Source: CAD feature listing. Evaluate the final solid. Frame: model axes, mm. Round coordinates to 2 decimals unless told otherwise and drop trailing zeros. Order: outer loops, then holes, each group sorted by start corner. A loop starts at its lowest first (then second) coordinate and runs counter-clockwise, first axis right, second up. Notation, with made-up numbers: (11, 8.5) -> (47, 8.5) arc R29 cw to (47, 42.5) -> close; hole circle Ø8 at (-12, -34). An arc over 180 degrees is marked (long way). Answer as CSV lines item,"result". Start each with the question number.
(1) Section query A-A (x = -82). Output: boundary loops of the cut face in (y, z), plus the area to 3 significant figures.
(2) Section query D-D (z = 1.5). Count the separate pieces of the cut face and the enclosed holes in it, plus the area to 3 significant figures.
(3) Section query C-C (x = -98). Output: boundary loops of the cut face in (y, z), plus the area to 3 significant figures.
(4) Contact query for flat-ended pins moving along their axis: P1, Ø1.8, axis at x = -69.58, y = -54.6, coming from the +Z side; P2, Ø3, axis at y = -96, z = 1, coming from the +X side; P3, Ø1, axis at x = -31.5, z = -1, coming from the +Y side; P4, Ø2, axis at x = -53.5, z = 0, coming from the +Y side. Output: stop coordinate, or through.
(5) Line query: line 1 along Y through (x, z) = (0, -0.8) (3 decimals); line 2 along X through (y, z) = (-65, -0.15); line 3 along Y through (x, z) = (-26.5, 1.15). Output: solid intervals per line, ascending. Write a range as from..to.
(6) Section query B-B (x = -54). Output: boundary loops of the cut face in (y, z).
```python
from build123d import *

# Parameters (mm, degrees)
SKETCH_1_R               = 18.5
SKETCH_1_R_2             = 1.525
SKETCH_1_R_3             = 3
EXTRUDE_1_DEPTH          = 2.5
SKETCH_4_R               = 1.525
CUT_EXTRUDE_3_DEPTH      = 10
PATTERN_CIRCULAR_2_COUNT = 6
SKETCH_5_R               = 1.525
CUT_EXTRUDE_4_DEPTH      = 31.54
CUT_EXTRUDE_5_DEPTH      = 31.54
EXTRUDE_2_DEPTH          = 5
EXTRUDE_3_DEPTH          = 5
FILLET_2_R               = 1.5
FILLET_2_2_R             = 3
CUT_EXTRUDE_7_DEPTH      = 5
FILLET_4_R               = 1.2
FILLET_5_R               = 2


with BuildPart() as part:
    # Sketch 1 → Extrude 1 (new body, symmetric)
    with BuildSketch(Plane.XY):
        with BuildLine():
            Line((-102.821191847, -92.640522116), (-2.926441218, -138.613082375))
            ThreePointArc((-2.926441218, -138.613082375), (3.8087152, -138.127288993), (6.999564642, -132.176086843))
            Line((6.999564642, -132.176086843), (5.524656378, 0.061619046))
            ThreePointArc((5.524656378, 0.061619046), (2.952791693, 4.66975869), (-2.312992999, 5.01753808))
            Line((-2.312992999, 5.01753808), (-102.837527006, -41.322427799))
            ThreePointArc((-102.837527006, -41.322427799), (-119.260909787, -66.986705315), (-102.821191847, -92.640522116))
        make_face()
        with Locations((-91.010911218, -66.977713005)):
            Circle(SKETCH_1_R, mode=Mode.SUBTRACT)
        Circle(SKETCH_1_R_2, mode=Mode.SUBTRACT)
        with Locations((0, -132.254156223)):
            Circle(SKETCH_1_R_3, mode=Mode.SUBTRACT)
    extrude(amount=EXTRUDE_1_DEPTH, both=True)

    # Sketch 4 → Cut-Extrude 3 (cut)
    with BuildSketch(Plane.XY.offset(2.5)):
        with Locations((-91.010911218, -42.227713005)):
            Circle(SKETCH_4_R)
    cut_extrude_3 = extrude(amount=-CUT_EXTRUDE_3_DEPTH, mode=Mode.SUBTRACT)

    # Pattern Circular 2: Cut-Extrude 3 ×6 about axis
    pattern_circular_2_axis = Axis((-91.010911218, -66.977713005, 0), (0, 0, 1))
    for i in range(1, PATTERN_CIRCULAR_2_COUNT):
        add(cut_extrude_3.rotate(pattern_circular_2_axis, i * 360 / PATTERN_CIRCULAR_2_COUNT), mode=Mode.SUBTRACT)

    # Sketch 5 → Cut-Extrude 4 (cut)
    with BuildSketch(Plane.XY.offset(2.5)):
        with Locations((-2.745656165, -29.87409199)):
            Circle(SKETCH_5_R)
        with Locations((-27.244550661, -12.559238006)):
            Circle(SKETCH_5_R)
    extrude(amount=-CUT_EXTRUDE_4_DEPTH, mode=Mode.SUBTRACT)

    # Sketch 6 → Cut-Extrude 5 (cut)
    with BuildSketch(Plane.XY.offset(2.5)):
        with BuildLine():
            Line((-79.067859687, -41.376423581), (-29.316651197, -18.44202924))
            Line((-29.316651197, -18.44202924), (-4.070575386, -36.284961557))
            Line((-4.070575386, -36.284961557), (-3.117843226, -121.705267485))
            ThreePointArc((-3.117843226, -121.705267485), (-5.985123886, -123.024947586), (-8.359603594, -125.104538908))
            Line((-8.359603594, -125.104538908), (-79.051563719, -92.57139401))
            ThreePointArc((-79.051563719, -92.57139401), (-62.760912649, -66.968720694), (-79.067859687, -41.376423581))
        make_face()
    extrude(amount=-CUT_EXTRUDE_5_DEPTH, mode=Mode.SUBTRACT)

    # Sketch 7 → Extrude 2 (add)
    with BuildSketch(Plane.XY.offset(2.5)):
        with BuildLine():
            Line((-73.548163223, -95.104113791), (-69.036338231, -97.180500639))
            Line((-69.036338231, -97.180500639), (-4.005429036, -42.12586983))
            Line((-4.005429036, -42.12586983), (-4.070575386, -36.284961557))
            Line((-4.070575386, -36.284961557), (-7.866276061, -33.602309776))
            Line((-7.866276061, -33.602309776), (-72.757541368, -88.538719222))
            ThreePointArc((-72.757541368, -88.538719222), (-75.770580222, -90.764154755), (-79.051563719, -92.57139401))
            Line((-79.051563719, -92.57139401), (-73.548163223, -95.104113791))
        make_face()
    extrude(amount=-EXTRUDE_2_DEPTH)

    # Sketch 8 → Extrude 3 (add)
    with BuildSketch(Plane(origin=(0, 0, -2.5), x_dir=(-1, 0, 0), z_dir=(0, 0, -1))):
        Polygon((7.967241055, -126.608441364), (39.55881203, -71.391285075), (33.804329575, -67.353372997), (1.891384262, -123.132241683), align=None)
    extrude(amount=-EXTRUDE_3_DEPTH)

    # Fillet 2
    fillet_2_edges = [part.edges().sort_by_distance(p)[0] for p in [
        (-69.036338231, -97.180500639, 0),
        (-39.237437692, -71.952997472, 0),
        (-33.804329575, -67.353372997, 0),
        (-4.005429036, -42.12586983, 0),
        (-7.866276061, -33.602309776, 0),
        (-79.067859687, -41.376423581, 0),
        (-29.316651197, -18.44202924, 0),
    ]]
    fillet(fillet_2_edges, radius=FILLET_2_R)

    # Fillet 2 2
    fillet_2_2_edges = [part.edges().sort_by_distance(p)[0] for p in [
        (-72.757541368, -88.538719222, 0),
    ]]
    fillet(fillet_2_2_edges, radius=FILLET_2_2_R)

    # Sketch 12 → Cut-Extrude 7 (cut)
    with BuildSketch(Plane.XY.offset(2.5)):
        Polygon((-3.462970797, -4.899778899), (-21.269732263, -13.108369239), (-5.257503766, -24.425181858), align=None)
    extrude(amount=-CUT_EXTRUDE_7_DEPTH, mode=Mode.SUBTRACT)

    # Fillet 4
    fillet_4_edges = [part.edges().sort_by_distance(p)[0] for p in [
        (-3.462970797, -4.899778899, 0),
        (-5.257503766, -24.425181858, 0),
        (-21.269732263, -13.108369239, 0),
    ]]
    fillet(fillet_4_edges, radius=FILLET_4_R)

    # Fillet 5
    fillet_5_edges = [part.edges().sort_by_distance(p)[0] for p in [
        (-8.994965293, -124.812139119, 0),
        (-3.125995679, -120.974332802, 0),
    ]]
    fillet(fillet_5_edges, radius=FILLET_5_R)


solid = part.part
```
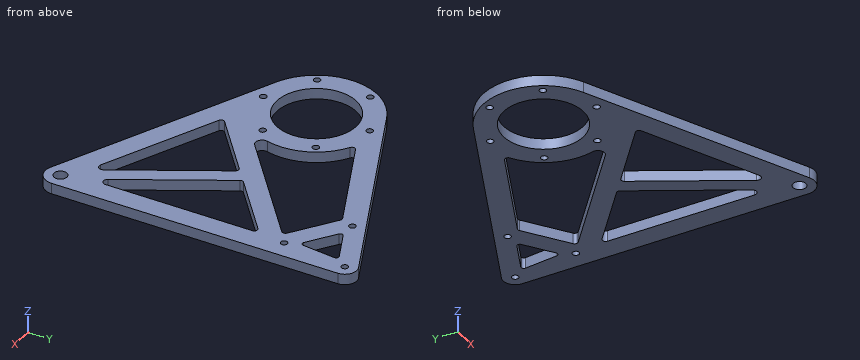
Answer block:
1,outline,"(-102.22, -2.5) -> (-83.13, -2.5) -> (-83.13, 2.5) -> (-102.22, 2.5) -> close; (-50.82, -2.5) -> (-31.72, -2.5) -> (-31.72, 2.5) -> (-50.82, 2.5) -> close"
1,area,"191 mm2"
2,separate pieces,"1"
2,enclosed holes,"15"
2,area,"6,120 mm2"
3,outline,"(-94.86, -2.5) -> (-84.11, -2.5) -> (-84.11, 2.5) -> (-94.86, 2.5) -> close; (-49.85, -2.5) -> (-39.09, -2.5) -> (-39.09, 2.5) -> (-49.85, 2.5) -> close"
3,area,"108 mm2"
4,P1,"through"
4,P2,"x = 6.61"
4,P3,"y = -8.21"
4,P4,"y = -18.12"
5,line 1,"-139.254..-135.254, -129.254..-1.525, 1.525..5.525"
5,line 2,"-119.19..-109.4, -72.62..-62.83, -44.95..-31.02, -3.75..6.25"
5,line 3,"-127.76..-116.76, -94.22..-80.12, -61.17..-49.38, -20.43..-13.89, -11.23..-6.13"
6,outline,"(-115.11, -2.5) -> (-104.1, -2.5) -> (-104.1, 2.5) -> (-115.11, 2.5) -> close; (-84.45, -2.5) -> (-72.66, -2.5) -> (-72.66, 2.5) -> (-84.45, 2.5) -> close; (-29.82, -2.5) -> (-18.81, -2.5) -> (-18.81, 2.5) -> (-29.82, 2.5) -> close"
